```python
from build123d import *

# Parameters (mm, degrees)
SKETCH1_R           = 3
BOSS_EXTRUDE1_DEPTH = 0.6


with BuildPart() as part:
    # Sweep1: sweep along a path in Sketch2
    with BuildLine(Plane.XY) as sweep1_path:
        Line((-17.5, 0), (-17.5, 42.5))
        ThreePointArc((-17.5, 42.5), (0, 60), (17.5, 42.5))
        Line((17.5, 42.5), (17.5, 0))
    # Sketch1 → Sweep1 (sweep)
    with BuildSketch(Plane(origin=(0, 0, 0), x_dir=(1, 0, 0), z_dir=(0, 1, 0))):
        with Locations((-17.5, 0)):
            Circle(SKETCH1_R)
    sweep(path=sweep1_path.line)

    # Sketch3 → Boss-Extrude1 (add)
    with BuildSketch(Plane(origin=(0, 10, 0), x_dir=(1, 0, 0), z_dir=(0, 1, 0))):
        with BuildLine():
            Line((-17.5, -4.5), (17.5, -4.5))
            ThreePointArc((17.5, -4.5), (22, 0), (17.5, 4.5))
            Line((17.5, 4.5), (-17.5, 4.5))
            ThreePointArc((-17.5, 4.5), (-22, 0), (-17.5, -4.5))
        make_face()
    extrude(amount=BOSS_EXTRUDE1_DEPTH)


solid = part.part
```
Could you check a few things on this model? Use its own coordinates, in mm. A direction names the side the tool comes from. Round coordinates to 2 decimals unless told otherwise and drop trailing zeros. Loops run counter-clockwise (first coordinate to the right, second up) from the corner with the lowest first, then second, coordinate; pieces in that order, holes last. Notation, with made-up numbers: (64.25, -17.5) - (103.25, -17.5) arc R20 cw to (103.25, -13.5) - close; hole circle Ø4 at (-13, -3.75). An arc over 180 degrees is marked (long way). Answer in a Markdown table with one row per item. Add a question column.
(1) I need wall thicknesses on line 1 along X through (y, z) = (5.5, 0.25); line 2 along X through (y, z) = (25.5, -2); line 3 along Y through (x, z) = (-10, 3.5). Which ranges of each line are inside material? Lowest first, please.
(2) If we section it at B-B (y = 22): Please give me the cut outline in (x, z), plus the area to 3 significant figures.
(3) If we section it at A-A (z = 0): Please give me the cut outline in (x, y), plus the area to 3 significant figures.
(4) For faces 4 (the face through (20.5, 26.3, -0.1)), 5 (the face through (20.5, 4.9, -0.1)), 6 (the face through (22, 10.3, 0.1)), which set-ups out of +Z, -Z, +X, -X, +Y, -Y let a thin tool reach every point of the face, with its end or its side?
(5) If we mould it in two halves opening along X, with no side actions, what happens to faces 1 (the face through (-22, 10.3, -0.1)), 2 (the face through (0, 10.6, 0)), 3 (the face through (18, 0, 0))? For each: pulls with the +X half, pulls with the -X half, needs draft (parallel to the pull), parting line crosses it, or undercut.
(6) I'm going to push flat-ended pins straight in: pin 1 (2 mm diameter, centred on y = 14, z = -2, fed in from +X); pin 2 (2 mm diameter, centred on y = 39.5, z = 1, fed in from -X); pin 3 (4 mm diameter, centred on x = -3, z = 0, fed in from -Y). Where does each tip first touch, or does it pass through?
Model answer:
| question | item | result |
|---|---|---|
| 1 | line 1 | x = -20.49 to -14.51, 14.51 to 20.49 |
| 1 | line 2 | x = -19.74 to -15.26, 15.26 to 19.74 |
| 1 | line 3 | y = 10 to 10.6 |
| 2 | outline | circle Ø6 at (-17.5, 0); circle Ø6 at (17.5, 0) |
| 2 | area | 56.5 mm² |
| 3 | outline | (-22, 10) - (-20.5, 10) - (-20.5, 0) - (-14.5, 0) - (-14.5, 10) - (14.5, 10) - (14.5, 0) - (20.5, 0) - (20.5, 10) - (22, 10) - (22, 10.6) - (20.5, 10.6) - (20.5, 42.5) arc R20.5 ccw to (-20.5, 42.5) - (-20.5, 10.6) - (-22, 10.6) - close; hole (-14.5, 10.6) - (14.5, 10.6) - (14.5, 42.5) arc R14.5 ccw to (-14.5, 42.5) - close |
| 3 | area | 859 mm² |
| 4 | face 4 | none |
| 4 | face 5 | -Y |
| 4 | face 6 | +X, +Y, -Y |
| 5 | face 1 | pulls with the -X half |
| 5 | face 2 | undercut |
| 5 | face 3 | needs draft |
| 6 | pin 1 | stops at x = 20.33 |
| 6 | pin 2 | stops at x = -20.5 |
| 6 | pin 3 | stops at y = 10 |
